For this review, take the finished solid that the model builds, in its own axes (mm). A direction names the side the tool comes from. Coordinates: 2 decimals unless noted, no trailing zeros. Loops run counter-clockwise (first coordinate to the right, second up) from the corner with the lowest first, then second, coordinate; pieces in that order, holes last. Notation, with made-up numbers: (11, -32) -> (66, -32) arc R15 ccw to (66, -10) -> close; hole circle Ø10 at (-37, 15.5). An arc over 180 degrees is marked (long way). Use a Markdown table: item, result.
from build123d import *

# Parameters (mm, degrees)
F1_DEPTH = 4.99999
F2_R     = 8.34999981
F2_R_2   = 3.048
F3_DEPTH = 16.9999914
F4_R     = 1.4581169527
F5_DEPTH = 25.4
F6_R     = 5.5000017
F7_DEPTH = 47.999904
F9_DEPTH = 29.99994


# Not quite as in the source:
# - ends of sketch curves that miss each other by under 0.0002 mm in the source are joined


with BuildPart() as f1:
    # F0 (on Top) → F1 (new body)
    with BuildSketch(Plane.XY):
        Polygon((10.0000054, 0), (5.0000027, 8.6602587144), (-5.0000027, 8.6602587144), (-10.0000054, 0), (-5.0000027, -8.6602587144), (5.0000027, -8.6602587144), align=None)
    extrude(amount=F1_DEPTH)

    # F2 (on face) → F3 (join)
    with BuildSketch(Plane.XY.offset(4.99999)):
        Circle(F2_R)
        Circle(F2_R_2, mode=Mode.SUBTRACT)
    extrude(amount=F3_DEPTH)

    # F4 (on face) → F5 (cut)
    with BuildSketch(Plane(origin=(-7.50000405, -4.3301293572, 0), x_dir=(0.5, -0.8660254038, 0), z_dir=(-0.8660254038, -0.5, 0))):
        with Locations((0, 14.2499814)):
            Circle(F4_R)
    extrude(amount=-F5_DEPTH, mode=Mode.SUBTRACT)

    # F6 (on face) → F7 (join)
    with BuildSketch(Plane(origin=(0, 0, 0), x_dir=(1, 0, 0), z_dir=(0, 0, -1))):
        Circle(F6_R)
    extrude(amount=F7_DEPTH)

    # F8 (on face) → F9 (cut)
    with BuildSketch(Plane(origin=(0, 0, -47.999904), x_dir=(1, 0, 0), z_dir=(0, 0, -1))):
        with BuildLine():
            Line((2.5, -4.8989813941), (2.5, 0))
            ThreePointArc((2.5, 0), (0, 2.499995), (-2.499995, 0))
            Line((-2.499995, 0), (-2.5, -4.8989813941))
            ThreePointArc((-2.5, -4.8989813941), (0, -5.5000017), (2.5, -4.8989813941))
        make_face()
    extrude(amount=-F9_DEPTH, mode=Mode.SUBTRACT)


solid = f1.part
(1) For line 1 along Y through (x, z) = (0, 18.5); line 2 along Z through (x, y) = (0, -2.25); line 3 along Y through (x, z) = (0, -23), list the stretches that pass through material, from the lowest coordinate up.
Found:
| item | result |
|---|---|
| line 1 | y = -8.35 to -3.05, 3.05 to 8.35 |
| line 2 | z = -18 to 5 |
| line 3 | y = -5.5 to -2.5 |
(2) For faces 1 (the face through (7.535, 4.27, 2.465)), 2 (the face through (-0.716, -5.453, -23.664)), 3 (the face through (0, 1, -18)), 4 (the face through (4.49, 7.04, 13.38)), list the 3-axis set-ups (+Z, -Z, +X, -X, +Y, -Y) from which the entire face can be reached by the end or side of a thin tool; tool diameter is ignored.
Found:
| item | result |
|---|---|
| face 1 | +Z, -Z, +X, +Y |
| face 2 | -Z |
| face 3 | -Z, +Y |
| face 4 | +Z |
(3) Take a section at A-A on x = 0. Write out the cut boundary in (y, z).
Found:
| item | result |
|---|---|
| outline | (-8.66, 0) -> (-5.5, 0) -> (-5.5, -48) -> (-2.5, -48) -> (-2.5, -18) -> (5.5, -18) -> (5.5, 0) -> (8.66, 0) -> (8.66, 5) -> (8.35, 5) -> (8.35, 22) -> (3.05, 22) -> (3.05, 5) -> (-3.05, 5) -> (-3.05, 22) -> (-8.35, 22) -> (-8.35, 5) -> (-8.66, 5) -> close |
(4) Take a section at C-C on z = -4.5. Write out the cut boundary in (x, y), plus the area to 3 significant figures.
Found:
| item | result |
|---|---|
| outline | circle Ø11 at (0, 0) |
| area | 95.0 mm^2 |
(5) Take a section at D-D on y = -6.25. Write out the cut boundary in (x, z).
Found:
| item | result |
|---|---|
| outline | (-6.39, 0) -> (6.39, 0) -> (6.39, 5) -> (5.54, 5) -> (5.54, 22) -> (-5.54, 22) -> (-5.54, 5) -> (-6.39, 5) -> close |
(6) For pin 1 Ø5.5 at (x, y) = (0, 0) entering from -Z; pin 2 Ø6 at (x, y) = (7.5, 4.5) entering from -Z; pin 3 Ø8 at (y, z) = (3.5, -35.5) entering from -X; pin 4 Ø8 at (y, z) = (-5, -18.5) entering from -X, all flat-tipped, find the tip position at first contact; note any pin that passes through.
Found:
| item | result |
|---|---|
| pin 1 | stops at z = -48 |
| pin 2 | stops at z = 0 |
| pin 3 | stops at x = -5.5 |
| pin 4 | stops at x = -5.41 |
(7) Take a section at B-B on y = 6.75. Write out the cut boundary in (x, z).
Found:
| item | result |
|---|---|
| outline | (-6.1, 0) -> (6.1, 0) -> (6.1, 5) -> (4.92, 5) -> (4.92, 22) -> (-4.92, 22) -> (-4.92, 5) -> (-6.1, 5) -> close |
(8) Mouldability with a two-part tool opening along Y and no side actions: class faces 5 (the face through (8, 3, 5)), 6 (the face through (0, 0, 5)), 7 (the face through (0, -8.66, 2)) as pulls with the +Y half, pulls with the -Y half, needs draft (parallel to the pull), parting line crosses it, or undercut.
Found:
| item | result |
|---|---|
| face 5 | needs draft |
| face 6 | undercut |
| face 7 | pulls with the -Y half |
